Geometry check sheet. Reference: the model listing, model coordinates, mm. Round coordinates to 2 decimals unless told otherwise and drop trailing zeros. Order: outer loops, then holes, each group sorted by start corner. A loop starts at its lowest first (then second) coordinate and runs counter-clockwise, first axis right, second up.
```python
from build123d import *

# Parameters (mm, degrees)
F0_W     = 779
F0_H     = 500
F1_DEPTH = 90
F2_SIZE  = 50
F3_W     = 708.4165965748
F3_H     = 398.4843355733
F4_DEPTH = 5
F6_D     = 5
F6_DEPTH = 10
F6_TIP   = 1.5021515476


with BuildPart() as f1:
    # F0 (on Front) → F1 (new body)
    with BuildSketch(Plane.XZ):
        Rectangle(F0_W, F0_H)
    extrude(amount=F1_DEPTH)

    # F2
    f2_edges = [f1.edges().sort_by_distance(p)[0] for p in [
        (389.5, 0, 0),
        (0, 0, 250),
        (-389.5, 0, 0),
        (0, 0, -250),
    ]]
    chamfer(f2_edges, length=F2_SIZE)

    # F3 (on face) → F4 (cut)
    with BuildSketch(Plane.XZ.offset(90)):
        Rectangle(F3_W, F3_H)
    extrude(amount=-F4_DEPTH, mode=Mode.SUBTRACT)

    # F6
    with Locations(Plane(origin=(0, 0, 0), x_dir=(-1, 0, 0), z_dir=(0, 1, 0))):
        with Locations((-100, 100), (100, 100), (-100, -100), (100, -100)):
            Hole(F6_D / 2, depth=F6_DEPTH)
            with Locations((0, 0, -(F6_DEPTH + F6_TIP / 2))):  # 118° drill point
                Cone(0, F6_D / 2, F6_TIP, mode=Mode.SUBTRACT)


solid = f1.part
```
(1) Sectioned sample at C-C, the plane y = -28. Record the cut outline in (x, z), and give its area (3 significant figures).
Returned:
outline: (-367.5, -228) - (367.5, -228) - (367.5, 228) - (-367.5, 228) - close
area: 335,000 mm2
(2) Material ranges on line 1 (Z direction, x = 100, y = -4); line 2 (Z direction, x = -100, y = -4.5); line 3 (X direction, y = -5.75, z = 100), recorded low to high.
Returned:
line 1: z = -204 to -102.5, -97.5 to 97.5, 102.5 to 204
line 2: z = -204.5 to -102.5, -97.5 to 97.5, 102.5 to 204.5
line 3: x = -345.25 to -102.5, -97.5 to 97.5, 102.5 to 345.25
(3) Draft check along Z on faces 1 (the flat face through (-5, -70, 250)), 2 (the flat face through (-5, -85, 3)), 3 (the flat face through (-5, -25, -225)), 4 (the flat face through (389.5, -70, -3)). Enter one of: released by +Z, released by -Z, zero draft, split by the parting line, or undercut.
Returned:
face 1: released by +Z
face 2: undercut
face 3: released by -Z
face 4: zero draft
(4) Sectioned sample at A-A, the plane z = -67. Record the cut outline in (x, y), and give its area (3 significant figures).
Returned:
outline: (-389.5, -90) - (-354.21, -90) - (-354.21, -85) - (354.21, -85) - (354.21, -90) - (389.5, -90) - (389.5, -50) - (339.5, 0) - (-339.5, 0) - (-389.5, -50) - close
area: 64,100 mm2
(5) Sectioned sample at B-B, the plane x = 175. Record the cut outline in (y, z), and give its area (3 significant figures).
Returned:
outline: (-90, -250) - (-50, -250) - (0, -200) - (0, 200) - (-50, 250) - (-90, 250) - (-90, 199.24) - (-85, 199.24) - (-85, -199.24) - (-90, -199.24) - close
area: 40,500 mm2
(6) Depth check by flat-ended pin: P1, Ø12, axis at y = -14.5, z = 53, coming from the -X side; P2, Ø3, axis at x = -100, z = -100, coming from the -Y side; P3, Ø10, axis at y = -12.5, z = 158.5, coming from the -X side. Enter the tip coordinate at first touch or a pass-through.
Returned:
P1: stops at x = -360
P2: stops at y = -85
P3: stops at x = -357
